```python
from build123d import *

# Parameters (mm, degrees)
SKETCH2_R           = 1.65
BOSS_EXTRUDE1_DEPTH = 7
SKETCH3_R           = 9.7
CUT_EXTRUDE1_DEPTH  = 5
SKETCH4_R           = 7.5
CUT_EXTRUDE2_DEPTH  = 5
CUT_EXTRUDE3_DEPTH  = 2.5
SKETCH6_R           = 7.5
SKETCH6_R_2         = 3.5
BOSS_EXTRUDE2_DEPTH = 1.8
SKETCH7_W           = 1.8
SKETCH7_H           = 2.5
CUT_EXTRUDE4_DEPTH  = 2.5
SKETCH8_R           = 2.1
CUT_EXTRUDE5_DEPTH  = 3


with BuildPart() as part:
    # Sketch2 → Boss-Extrude1 (new body)
    with BuildSketch(Plane.XY):
        with BuildLine():
            Line((-18, 9.5), (-7.331439149, 9.5))
            ThreePointArc((-7.331439149, 9.5), (0, 12), (7.331439149, 9.5))
            Line((7.331439149, 9.5), (18, 9.5))
            ThreePointArc((18, 9.5), (21.181980515, 8.181980515), (22.5, 5))
            Line((22.5, 5), (22.5, -5))
            ThreePointArc((22.5, -5), (21.181980515, -8.181980515), (18, -9.5))
            Line((18, -9.5), (7.331439149, -9.5))
            ThreePointArc((7.331439149, -9.5), (0, -12), (-7.331439149, -9.5))
            Line((-7.331439149, -9.5), (-18, -9.5))
            ThreePointArc((-18, -9.5), (-21.181980515, -8.181980515), (-22.5, -5))
            Line((-22.5, -5), (-22.5, 5))
            ThreePointArc((-22.5, 5), (-21.181980515, 8.181980515), (-18, 9.5))
        make_face()
        with Locations((-18, 5)):
            Circle(SKETCH2_R, mode=Mode.SUBTRACT)
        with Locations((18, 5)):
            Circle(SKETCH2_R, mode=Mode.SUBTRACT)
        with Locations((18, -5)):
            Circle(SKETCH2_R, mode=Mode.SUBTRACT)
        with Locations((-18, -5)):
            Circle(SKETCH2_R, mode=Mode.SUBTRACT)
    extrude(amount=BOSS_EXTRUDE1_DEPTH)

    # Sketch3 → Cut-Extrude1 (cut)
    with BuildSketch(Plane.XY):
        Circle(SKETCH3_R)
    extrude(amount=CUT_EXTRUDE1_DEPTH, mode=Mode.SUBTRACT)

    # Sketch4 → Cut-Extrude2 (cut)
    with BuildSketch(Plane(origin=(0, 0, 5), x_dir=(-1, 0, 0), z_dir=(0, 0, -1))):
        Circle(SKETCH4_R)
    extrude(amount=-CUT_EXTRUDE2_DEPTH, mode=Mode.SUBTRACT)

    # Sketch5 → Cut-Extrude3 (cut)
    with BuildSketch(Plane.XY.offset(7)):
        Polygon((-18, 8.348631561), (-20.9, 6.674315781), (-20.9, 3.325684219), (-18, 1.651368439), (-15.1, 3.325684219), (-15.1, 6.674315781), align=None)
        Polygon((15.1, 6.674315781), (18, 8.348631561), (20.9, 6.674315781), (20.9, 3.325684219), (18, 1.651368439), (15.1, 3.325684219), align=None)
        Polygon((15.1, -3.325684219), (15.1, -6.674315781), (18, -8.348631561), (20.9, -6.674315781), (20.9, -3.325684219), (18, -1.651368439), align=None)
        Polygon((-15.1, -6.674315781), (-18, -8.348631561), (-20.9, -6.674315781), (-20.9, -3.325684219), (-18, -1.651368439), (-15.1, -3.325684219), align=None)
    extrude(amount=-CUT_EXTRUDE3_DEPTH, mode=Mode.SUBTRACT)

    # Sketch6 → Boss-Extrude2 (add)
    with BuildSketch(Plane.XY.offset(7)):
        Circle(SKETCH6_R)
        Circle(SKETCH6_R_2, mode=Mode.SUBTRACT)
    extrude(amount=-BOSS_EXTRUDE2_DEPTH)

    # Sketch7 → Cut-Extrude4 (cut)
    with BuildSketch(Plane.XY.offset(7)):
        with Locations((8, 0)):
            Rectangle(SKETCH7_W, SKETCH7_H)
    extrude(amount=-CUT_EXTRUDE4_DEPTH, mode=Mode.SUBTRACT)

    # Sketch8 → Cut-Extrude5 (cut)
    with BuildSketch(Plane.XY.offset(7)):
        with Locations((-14, 0)):
            Circle(SKETCH8_R)
        with Locations((14, 0)):
            Circle(SKETCH8_R)
    extrude(amount=-CUT_EXTRUDE5_DEPTH, mode=Mode.SUBTRACT)


solid = part.part
```
Build history of the part. All positions in model axes, mm. A direction names the side the tool comes from. Coordinates: 2 decimals unless noted, no trailing zeros. Order: outer loops, then holes, each group sorted by start corner. A loop starts at its lowest first (then second) coordinate and runs counter-clockwise, first axis right, second up. Notation, with made-up numbers: (-17, 86) -> (-4, 86) arc R18 ccw to (-4, 117) -> close; hole circle Ø10 at (27, 79). An arc over 180 degrees is marked (long way). Answer in a Markdown table with one row per item. Add a question column.
Q1. Band-saw the part on D-D, the plane x = 8. List the corners of the cut face in (y, z).
Q2. Mould opens along X. For faces 5 (the face through (-19.3, 3.6, 4.5)), 6 (the face through (-21.147, -8.217, 3.451)), 7 (the face through (15.1, -5, 6)), 8 (the face through (0, -12, 3)) say: +X half, -X half, draft (parallel to the pull), parting line (faces both ways), or undercut.
Q3. Drop flat-ended pins along their axis: pin 1 (3 mm diameter, centred on x = 12, y = 8, fed in from -Z); pin 2 (2 mm diameter, centred on x = -13, y = 0, fed in from +Z); pin 3 (4.5 mm diameter, centred on x = 0.5, y = 2, fed in from -Z); pin 4 (2 mm diameter, centred on x = -16.5, z = 1, fed in from -Y). Give the stop position or say it passes through.
Q4. Which spindle directions (+Z, -Z, +X, -X, +Y, -Y) get a long thin tool onto all of the face, cutting with end or side? Do faces 1 (the face through (8, -1.25, 6)), 2 (the face through (13, -9.5, 3)), 3 (the face through (-22.5, 0, 3)), 4 (the face through (16.53, -7.5, 5.77)). Say none if no direction does.
Q5. Band-saw the part on C-C, the plane x = 14. List the corners of the cut face in (y, z), then the cut area to 3 significant figures.
Q6. Band-saw the part on A-A, the plane z = 1.5. List the corners of the cut face in (x, y), then the cut area to 3 significant figures.
Q7. Wall check: line 1 along X through (y, z) = (-4.5, 6.5); line 2 along Y through (x, z) = (-18, 1.9); line 3 along X through (y, z) = (2, 2.25). Give the ranges that are in metal, low to high. Write a range as [from, to].
Q8. Band-saw the part on B-B, the plane y = -4.25. List the corners of the cut face in (x, z).
Answers follow:
| question | item | result |
|---|---|---|
| 1 | outline | (-9.5, 0) -> (-5.49, 0) -> (-5.49, 5) -> (-1.25, 5) -> (-1.25, 7) -> (-9.5, 7) -> close; (1.25, 5) -> (5.49, 5) -> (5.49, 0) -> (9.5, 0) -> (9.5, 7) -> (1.25, 7) -> close |
| 2 | face 5 | undercut |
| 2 | face 6 | -X half |
| 2 | face 7 | undercut |
| 2 | face 8 | parting line |
| 3 | pin 1 | z = 0 |
| 3 | pin 2 | z = 4 |
| 3 | pin 3 | z = 5.2 |
| 3 | pin 4 | y = -9.5 |
| 4 | face 1 | +Z, -Z |
| 4 | face 2 | +Z, -Z, +X, -Y |
| 4 | face 3 | +Z, -Z, -X, +Y, -Y |
| 4 | face 4 | +Z |
| 5 | outline | (-9.5, 0) -> (9.5, 0) -> (9.5, 7) -> (2.1, 7) -> (2.1, 4) -> (-2.1, 4) -> (-2.1, 7) -> (-9.5, 7) -> close |
| 5 | area | 120 mm^2 |
| 6 | outline | (-22.5, -5) arc R4.5 ccw to (-18, -9.5) -> (-7.33, -9.5) arc R12 ccw to (7.33, -9.5) -> (18, -9.5) arc R4.5 ccw to (22.5, -5) -> (22.5, 5) arc R4.5 ccw to (18, 9.5) -> (7.33, 9.5) arc R12 ccw to (-7.33, 9.5) -> (-18, 9.5) arc R4.5 ccw to (-22.5, 5) -> close; hole circle Ø3.3 at (-18, -5); hole circle Ø3.3 at (-18, 5); hole circle Ø19.4 at (0, 0); hole circle Ø3.3 at (18, -5); hole circle Ø3.3 at (18, 5) |
| 6 | area | 558 mm^2 |
| 7 | line 1 | [-22.5, -20.9], [-15.1, 15.1], [20.9, 22.5] |
| 7 | line 2 | [-9.5, -6.65], [-3.35, 3.35], [6.65, 9.5] |
| 7 | line 3 | [-22.5, -9.49], [9.49, 22.5] |
| 8 | outline | (-22.5, 0) -> (-19.47, 0) -> (-19.47, 4.5) -> (-20.9, 4.5) -> (-20.9, 7) -> (-22.5, 7) -> close; (-16.53, 0) -> (-8.72, 0) -> (-8.72, 5) -> (-6.18, 5) -> (-6.18, 5.2) -> (6.18, 5.2) -> (6.18, 5) -> (8.72, 5) -> (8.72, 0) -> (16.53, 0) -> (16.53, 4.5) -> (15.1, 4.5) -> (15.1, 7) -> (-15.1, 7) -> (-15.1, 4.5) -> (-16.53, 4.5) -> close; (19.47, 0) -> (22.5, 0) -> (22.5, 7) -> (20.9, 7) -> (20.9, 4.5) -> (19.47, 4.5) -> close |
